For this review, take the finished solid that the model builds, in its own axes (mm). A direction names the side the tool comes from. Give positions to 0.01 mm unless a question says otherwise; leave off trailing zeros. Loops run counter-clockwise (first coordinate to the right, second up) from the corner with the lowest first, then second, coordinate; pieces in that order, holes last.
```python
from build123d import *

# Parameters (mm, degrees)
SKETCH_1_W                       = 300
SKETCH_1_H                       = 300
EXTRUDE_1_DEPTH                  = 1456
SKETCH_2_W                       = 240
SKETCH_2_H                       = 240
CUT_EXTRUDE_1_DEPTH              = 1517.553988488
SKETCH_4_W                       = 1256
SKETCH_4_H                       = 100
CUT_EXTRUDE_2_DEPTH              = 1517.553988488
SKETCH_5_W                       = 470
SKETCH_5_H                       = 470
EXTRUDE_2_DEPTH                  = 22
SKETCH_6_W                       = 470
SKETCH_6_H                       = 470
EXTRUDE_3_DEPTH                  = 22
SKETCH_7_R                       = 11
CUT_EXTRUDE_3_DEPTH              = 1596.760007019
SKETCH_8_W                       = 300
SKETCH_8_H                       = 300
EXTRUDE_4_DEPTH                  = 10
SKETCH_9_W                       = 300
SKETCH_9_H                       = 300
EXTRUDE_5_DEPTH                  = 10
SKETCH_10_W                      = 300
SKETCH_10_H                      = 300
EXTRUDE_6_DEPTH                  = 10
SKETCH_11_W                      = 300
SKETCH_11_H                      = 300
EXTRUDE_7_DEPTH                  = 10
SKETCH_12_R                      = 11
CUT_EXTRUDE_4_DEPTH              = 1578.572185353
PATTERN_LINEAR_1_COUNT           = 2
PATTERN_LINEAR_1_PITCH           = 140
PATTERN_LINEAR_1_COUNT_DIR2      = 2
PATTERN_LINEAR_1_PITCH_DIR2      = 204
PATTERN_LINEAR_2_COUNT           = 2
PATTERN_LINEAR_2_PITCH           = 500
PATTERN_LINEAR_2_COPY_1_SKETCH_R = 11
PATTERN_LINEAR_2_COPY_1_DEPTH    = 1578.572185353
PATTERN_LINEAR_2_COPY_2_SKETCH_R = 11
PATTERN_LINEAR_2_COPY_2_DEPTH    = 1578.572185353
PATTERN_LINEAR_2_COPY_3_SKETCH_R = 11
PATTERN_LINEAR_2_COPY_3_DEPTH    = 1578.572185353
SKETCH_13_R                      = 11
CUT_EXTRUDE_5_DEPTH              = 1578.572185353
PATTERN_LINEAR_3_COUNT           = 2
PATTERN_LINEAR_3_PITCH           = 140
PATTERN_LINEAR_3_COUNT_DIR2      = 2
PATTERN_LINEAR_3_PITCH_DIR2      = 204
PATTERN_LINEAR_4_COUNT           = 2
PATTERN_LINEAR_4_PITCH           = 500
PATTERN_LINEAR_4_COPY_1_SKETCH_R = 11
PATTERN_LINEAR_4_COPY_1_DEPTH    = 1578.572185353
PATTERN_LINEAR_4_COPY_2_SKETCH_R = 11
PATTERN_LINEAR_4_COPY_2_DEPTH    = 1578.572185353
PATTERN_LINEAR_4_COPY_3_SKETCH_R = 11
PATTERN_LINEAR_4_COPY_3_DEPTH    = 1578.572185353
SKETCH_14_R                      = 40
CUT_EXTRUDE_6_DEPTH              = 1596.760007019


with BuildPart() as part:
    # 草图1 → 拉伸1 (new body)
    with BuildSketch(Plane.XY):
        with Locations((150, 150)):
            Rectangle(SKETCH_1_W, SKETCH_1_H)
    extrude(amount=EXTRUDE_1_DEPTH)

    # 草图2 → 切除-拉伸1 (cut, through all)
    with BuildSketch(Plane.XY.offset(1456)):
        with Locations((150, 150)):
            Rectangle(SKETCH_2_W, SKETCH_2_H)
    extrude(amount=-CUT_EXTRUDE_1_DEPTH, mode=Mode.SUBTRACT)

    # 草图4 → 切除-拉伸2 (cut, through all)
    with BuildSketch(Plane.ZY):
        with Locations((728, 150)):
            Rectangle(SKETCH_4_W, SKETCH_4_H)
    extrude(amount=-CUT_EXTRUDE_2_DEPTH, mode=Mode.SUBTRACT)

    # 草图5 → 拉伸2 (add)
    with BuildSketch(Plane.XY.offset(1456)):
        with Locations((150, 150)):
            Rectangle(SKETCH_5_W, SKETCH_5_H)
    extrude(amount=EXTRUDE_2_DEPTH)

    # 草图6 → 拉伸3 (add)
    with BuildSketch(Plane(origin=(0, 0, 0), x_dir=(-1, 0, 0), z_dir=(0, 0, -1))):
        with Locations((-150, 150)):
            Rectangle(SKETCH_6_W, SKETCH_6_H)
    extrude(amount=EXTRUDE_3_DEPTH)

    # 草图7 → 切除-拉伸3 (cut, through all)
    with BuildSketch(Plane.XY.offset(1478)):
        with Locations((-40, -40)):
            Circle(SKETCH_7_R)
        with Locations((40, -40)):
            Circle(SKETCH_7_R)
        with Locations((150, -40)):
            Circle(SKETCH_7_R)
        with Locations((260, -40)):
            Circle(SKETCH_7_R)
        with Locations((340, -40)):
            Circle(SKETCH_7_R)
        with Locations((-40, 340)):
            Circle(SKETCH_7_R)
        with Locations((40, 340)):
            Circle(SKETCH_7_R)
        with Locations((150, 340)):
            Circle(SKETCH_7_R)
        with Locations((260, 340)):
            Circle(SKETCH_7_R)
        with Locations((340, 340)):
            Circle(SKETCH_7_R)
        with Locations((-40, 40)):
            Circle(SKETCH_7_R)
        with Locations((-40, 260)):
            Circle(SKETCH_7_R)
        with Locations((340, 40)):
            Circle(SKETCH_7_R)
        with Locations((340, 260)):
            Circle(SKETCH_7_R)
    extrude(amount=-CUT_EXTRUDE_3_DEPTH, mode=Mode.SUBTRACT)

    # 草图8 → 拉伸4 (add)
    with BuildSketch(Plane(origin=(0, 300, 0), x_dir=(1, 0, 0), z_dir=(0, 1, 0))):
        with Locations((150, -478)):
            Rectangle(SKETCH_8_W, SKETCH_8_H)
        with Locations((150, -978)):
            Rectangle(SKETCH_8_W, SKETCH_8_H)
    extrude(amount=EXTRUDE_4_DEPTH)

    # 草图9 → 拉伸5 (add)
    with BuildSketch(Plane.XZ):
        with Locations((150, 478)):
            Rectangle(SKETCH_9_W, SKETCH_9_H)
        with Locations((150, 978)):
            Rectangle(SKETCH_9_W, SKETCH_9_H)
    extrude(amount=EXTRUDE_5_DEPTH)

    # 草图10 → 拉伸6 (add)
    with BuildSketch(Plane(origin=(300, 0, 0), x_dir=(0, 0, -1), z_dir=(1, 0, 0))):
        with Locations((-478, 150)):
            Rectangle(SKETCH_10_W, SKETCH_10_H)
        with Locations((-978, 150)):
            Rectangle(SKETCH_10_W, SKETCH_10_H)
    extrude(amount=EXTRUDE_6_DEPTH)

    # 草图11 → 拉伸7 (add)
    with BuildSketch(Plane.ZY):
        with Locations((478, 150)):
            Rectangle(SKETCH_11_W, SKETCH_11_H)
        with Locations((978, 150)):
            Rectangle(SKETCH_11_W, SKETCH_11_H)
    extrude(amount=EXTRUDE_7_DEPTH)

    # 草图12 → 切除-拉伸4 (cut, through all)
    with BuildSketch(Plane.ZY.offset(10)):
        with Locations((1048, 252)):
            Circle(SKETCH_12_R)
    cut_extrude_4 = extrude(amount=-CUT_EXTRUDE_4_DEPTH, mode=Mode.SUBTRACT)

    # 阵列(线性)1: Cut-Extrude 4 2 × 2
    with Locations(*[(0, -j * PATTERN_LINEAR_1_PITCH_DIR2, -i * PATTERN_LINEAR_1_PITCH) for i in range(PATTERN_LINEAR_1_COUNT) for j in range(PATTERN_LINEAR_1_COUNT_DIR2) if (i, j) != (0, 0)]):
        add(cut_extrude_4, mode=Mode.SUBTRACT)

    # 阵列(线性)2: 切除-拉伸4 ×2
    with Locations(*[(0, 0, -i * PATTERN_LINEAR_2_PITCH) for i in range(1, PATTERN_LINEAR_2_COUNT)]):
        add(cut_extrude_4, mode=Mode.SUBTRACT)

    # 阵列(线性)2 copy 1 sketch → 阵列(线性)2 copy 1 (cut, through all)
    with BuildSketch(Plane(origin=(-10, -204, -500), x_dir=(0, 0, 1), z_dir=(-1, 0, 0))):
        with Locations((1048, 252)):
            Circle(PATTERN_LINEAR_2_COPY_1_SKETCH_R)
    extrude(amount=-PATTERN_LINEAR_2_COPY_1_DEPTH, mode=Mode.SUBTRACT)

    # 阵列(线性)2 copy 2 sketch → 阵列(线性)2 copy 2 (cut, through all)
    with BuildSketch(Plane(origin=(-10, 0, -640), x_dir=(0, 0, 1), z_dir=(-1, 0, 0))):
        with Locations((1048, 252)):
            Circle(PATTERN_LINEAR_2_COPY_2_SKETCH_R)
    extrude(amount=-PATTERN_LINEAR_2_COPY_2_DEPTH, mode=Mode.SUBTRACT)

    # 阵列(线性)2 copy 3 sketch → 阵列(线性)2 copy 3 (cut, through all)
    with BuildSketch(Plane(origin=(-10, -204, -640), x_dir=(0, 0, 1), z_dir=(-1, 0, 0))):
        with Locations((1048, 252)):
            Circle(PATTERN_LINEAR_2_COPY_3_SKETCH_R)
    extrude(amount=-PATTERN_LINEAR_2_COPY_3_DEPTH, mode=Mode.SUBTRACT)

    # 草图13 → 切除-拉伸5 (cut, through all)
    with BuildSketch(Plane.XZ.offset(10)):
        with Locations(Location((48, 1048, 0), (0, 0, 270))):
            Circle(SKETCH_13_R)
    cut_extrude_5 = extrude(amount=-CUT_EXTRUDE_5_DEPTH, mode=Mode.SUBTRACT)

    # 阵列(线性)3: Cut-Extrude 5 2 × 2
    with Locations(*[(j * PATTERN_LINEAR_3_PITCH_DIR2, 0, -i * PATTERN_LINEAR_3_PITCH) for i in range(PATTERN_LINEAR_3_COUNT) for j in range(PATTERN_LINEAR_3_COUNT_DIR2) if (i, j) != (0, 0)]):
        add(cut_extrude_5, mode=Mode.SUBTRACT)

    # 阵列(线性)4: 切除-拉伸5 ×2
    with Locations(*[(0, 0, -i * PATTERN_LINEAR_4_PITCH) for i in range(1, PATTERN_LINEAR_4_COUNT)]):
        add(cut_extrude_5, mode=Mode.SUBTRACT)

    # 阵列(线性)4 copy 1 sketch → 阵列(线性)4 copy 1 (cut, through all)
    with BuildSketch(Plane(origin=(204, -10, -500), x_dir=(1, 0, 0), z_dir=(0, -1, 0))):
        with Locations(Location((48, 1048, 0), (0, 0, 270))):
            Circle(PATTERN_LINEAR_4_COPY_1_SKETCH_R)
    extrude(amount=-PATTERN_LINEAR_4_COPY_1_DEPTH, mode=Mode.SUBTRACT)

    # 阵列(线性)4 copy 2 sketch → 阵列(线性)4 copy 2 (cut, through all)
    with BuildSketch(Plane(origin=(0, -10, -640), x_dir=(1, 0, 0), z_dir=(0, -1, 0))):
        with Locations(Location((48, 1048, 0), (0, 0, 270))):
            Circle(PATTERN_LINEAR_4_COPY_2_SKETCH_R)
    extrude(amount=-PATTERN_LINEAR_4_COPY_2_DEPTH, mode=Mode.SUBTRACT)

    # 阵列(线性)4 copy 3 sketch → 阵列(线性)4 copy 3 (cut, through all)
    with BuildSketch(Plane(origin=(204, -10, -640), x_dir=(1, 0, 0), z_dir=(0, -1, 0))):
        with Locations(Location((48, 1048, 0), (0, 0, 270))):
            Circle(PATTERN_LINEAR_4_COPY_3_SKETCH_R)
    extrude(amount=-PATTERN_LINEAR_4_COPY_3_DEPTH, mode=Mode.SUBTRACT)

    # 草图14 → 切除-拉伸6 (cut, through all)
    with BuildSketch(Plane.XY.offset(1478)):
        with Locations((150, 150)):
            Circle(SKETCH_14_R)
    extrude(amount=-CUT_EXTRUDE_6_DEPTH, mode=Mode.SUBTRACT)


solid = part.part
```
Item 1: Tool access review of faces 4 (the flat face through (148, -10, 480)), 5 (the flat face through (148, 310, 476)), 6 (the flat face through (15, 149, 1356)), 7 (the flat face through (285, 200, 719)): name each direction out of +Z, -Z, +X, -X, +Y, -Y from which nothing blocks a thin tool from reaching the whole face with its end or side.
Answer:
face 4: +X, -X, -Y
face 5: +X, -X, +Y
face 6: +X, -X
face 7: none
Item 2: For L1, parallel to X at y = 296.5, z = 548; L2, parallel to Y at x = 286, z = 908; L3, parallel to Z at x = -6.5, y = 35.5, list the stretches that pass through material, from the lowest coordinate up.
Answer:
L1: x = -10 to 37, 59 to 241, 263 to 310
L2: y = -10 to 37, 59 to 100, 200 to 241, 263 to 310
L3: z = -22 to 0, 328 to 628, 828 to 1128, 1456 to 1478
Item 3: Take a section at A-A on z = 1196. Give the boundary of the cut face in (x, y), and give its area (3 significant figures).
Answer:
outline: (0, 0) - (300, 0) - (300, 100) - (270, 100) - (270, 30) - (30, 30) - (30, 100) - (0, 100) - close; (0, 200) - (30, 200) - (30, 270) - (270, 270) - (270, 200) - (300, 200) - (300, 300) - (0, 300) - close
area: 26,400 mm2
Item 4: The part is to be moulded in two halves that separate along Y. For faces 1 (the flat face through (0, 249, 727)), 2 (the flat face through (270, 95, 738)), 3 (the flat face through (148, 0, 1290)), say which applies: released by +Y, released by -Y, zero draft, split by the parting line, or undercut.
Answer:
face 1: zero draft
face 2: undercut
face 3: released by -Y
Item 5: Clearance check with flat-ended pins moving along their axes: pin 1 Ø1 at (y, z) = (6.5, 1067) entering from -X; pin 2 Ø12 at (x, z) = (149.5, 496) entering from +Y; pin 3 Ø12 at (x, z) = (30.5, 636) entering from -Y. State where each tip first meets the part, or that it passes through.
Answer:
pin 1: stops at x = -10
pin 2: stops at y = 310
pin 3: stops at y = 0
Item 6: Take a section at C-C on z = 610. Give the boundary of the cut face in (x, y), and give its area (3 significant figures).
Answer:
outline: (-10, 0) - (0, 0) - (0, -10) - (300, -10) - (300, 0) - (310, 0) - (310, 300) - (300, 300) - (300, 310) - (0, 310) - (0, 300) - (-10, 300) - close; hole (0, 100) - (30, 100) - (30, 30) - (270, 30) - (270, 100) - (300, 100) - (300, 200) - (270, 200) - (270, 270) - (30, 270) - (30, 200) - (0, 200) - close
area: 38,400 mm2
